from build123d import *

# Parameters (mm, degrees)
F0_R     = 16.51
F1_DEPTH = 50.8
F2_R     = 94.742
F2_R_2   = 75.438
F3_DEPTH = 12.7
F4_R     = 75.438
F5_DEPTH = 31.75
F6_R     = 112.776
F6_R_2   = 69.85
F7_DEPTH = 63.5
F8_R     = 69.85
F9_DEPTH = 76.2


with BuildPart() as f1:
    # F0 (on Top) → F1 (new body)
    with BuildSketch(Plane.XY):
        with BuildLine():
            Line((226.06, 0), (302.641, 0))
            ThreePointArc((302.641, 0), (301.183701, 29.664005), (296.825838, 59.04233))
            Line((296.825838, 59.04233), (34.253926, 6.813529))
            ThreePointArc((34.253926, 6.813529), (34.756827, 3.423249), (34.925, 0))
            Line((34.925, 0), (193.04, 0))
            ThreePointArc((193.04, 0), (209.55, 16.51), (226.06, 0))
        make_face()
        with BuildLine():
            ThreePointArc((0, 302.641), (-213.999503, -213.999503), (302.641, 0))
            Line((302.641, 0), (226.06, 0))
            ThreePointArc((226.06, 0), (209.55, -16.51), (193.04, 0))
            Line((193.04, 0), (34.925, 0))
            ThreePointArc((34.925, 0), (-24.695704, -24.695704), (0, 34.925))
            Line((0, 34.925), (0, 148.59))
            ThreePointArc((0, 148.59), (-16.51, 165.1), (0, 181.61))
            Line((0, 181.61), (0, 232.41))
            ThreePointArc((0, 232.41), (-16.51, 248.92), (0, 265.43))
            Line((0, 265.43), (0, 302.641))
        make_face()
        with Locations((-95.25756, -229.972093)):
            Circle(F0_R, mode=Mode.SUBTRACT)
        with Locations((-63.181035, -152.532511)):
            Circle(F0_R, mode=Mode.SUBTRACT)
        with Locations((-193.598956, -80.191313)):
            Circle(F0_R, mode=Mode.SUBTRACT)
        with Locations((0, -248.92)):
            Circle(F0_R, mode=Mode.SUBTRACT)
        with Locations((95.25756, -229.972093)):
            Circle(F0_R, mode=Mode.SUBTRACT)
        with Locations((0, -165.1)):
            Circle(F0_R, mode=Mode.SUBTRACT)
        with Locations((63.181035, -152.532511)):
            Circle(F0_R, mode=Mode.SUBTRACT)
        with Locations((193.598956, -80.191313)):
            Circle(F0_R, mode=Mode.SUBTRACT)
        with Locations((-209.55, 0)):
            Circle(F0_R, mode=Mode.SUBTRACT)
        with Locations((-193.598956, 80.191313)):
            Circle(F0_R, mode=Mode.SUBTRACT)
        with Locations((-63.181035, 152.532511)):
            Circle(F0_R, mode=Mode.SUBTRACT)
        with Locations((-95.25756, 229.972093)):
            Circle(F0_R, mode=Mode.SUBTRACT)
        with BuildLine():
            Line((34.253926, 6.813529), (296.825838, 59.04233))
            ThreePointArc((296.825838, 59.04233), (213.999503, 213.999503), (59.04233, 296.825838))
            Line((59.04233, 296.825838), (6.813529, 34.253926))
            ThreePointArc((6.813529, 34.253926), (24.695704, 24.695704), (34.253926, 6.813529))
        make_face()
        with Locations((193.598956, 80.191313)):
            Circle(F0_R, mode=Mode.SUBTRACT)
        with Locations((63.181035, 152.532511)):
            Circle(F0_R, mode=Mode.SUBTRACT)
        with Locations((95.25756, 229.972093)):
            Circle(F0_R, mode=Mode.SUBTRACT)
        with BuildLine():
            ThreePointArc((59.04233, 296.825838), (29.664005, 301.183701), (0, 302.641))
            Line((0, 302.641), (0, 265.43))
            ThreePointArc((0, 265.43), (11.674333, 260.594333), (16.51, 248.92))
            ThreePointArc((16.51, 248.92), (11.674333, 237.245667), (0, 232.41))
            Line((0, 232.41), (0, 181.61))
            ThreePointArc((0, 181.61), (11.674333, 176.774333), (16.51, 165.1))
            ThreePointArc((16.51, 165.1), (11.674333, 153.425667), (0, 148.59))
            Line((0, 148.59), (0, 34.925))
            ThreePointArc((0, 34.925), (3.423249, 34.756827), (6.813529, 34.253926))
            Line((6.813529, 34.253926), (59.04233, 296.825838))
        make_face()
    extrude(amount=F1_DEPTH)

    # F2 (on face) → F3 (join)
    with BuildSketch(Plane.XY.offset(50.8)):
        Circle(F2_R)
        Circle(F2_R_2, mode=Mode.SUBTRACT)
    extrude(amount=F3_DEPTH)

    # F4 (on face) → F5 (cut, symmetric)
    with BuildSketch(Plane.XY.offset(63.5)):
        Circle(F4_R)
    extrude(amount=F5_DEPTH, both=True, mode=Mode.SUBTRACT)

    # F6 (on face) → F7 (join)
    with BuildSketch(Plane(origin=(0, 0, 0), x_dir=(1, 0, 0), z_dir=(0, 0, -1))):
        Circle(F6_R)
        Circle(F6_R_2, mode=Mode.SUBTRACT)
    extrude(amount=F7_DEPTH)

    # F8 (on face) → F9 (cut)
    with BuildSketch(Plane(origin=(0, 0, -63.5), x_dir=(1, 0, 0), z_dir=(0, 0, -1))):
        Circle(F8_R)
    extrude(amount=-F9_DEPTH, mode=Mode.SUBTRACT)


solid = f1.part
Can you work these out from the model? Positions are in its coordinate system, mm. A direction names the side the tool comes from. Coordinates: 2 decimals unless noted, no trailing zeros. Order: outer loops, then holes, each group sorted by start corner. A loop starts at its lowest first (then second) coordinate and runs counter-clockwise, first axis right, second up. Notation, with made-up numbers: M 64.25,21 L 72.25,21 A24 ccw 72.25,51 Z; hole C 44.25,20.25 d9. An arc over 180 degrees is marked long. Answer as CSV lines item,"result".
(1) If we mould it in two halves opening along X, with no side actions, what happens to faces 1 (the cylindrical face through (-69.83, 64.03, 57.06)), 2 (the cylindrical face through (193.056, -0.726, 25.044)), 3 (the flat face through (-71, -63, 50.8))? For each: released by +X, released by -X, zero draft, split by the parting line, or undercut.
Geometry check:
face 1,"split by the parting line"
face 2,"undercut"
face 3,"zero draft"
(2) Suppose I cut it at D-D on y = 124.5. Please give me the cut outline in (x, z).
Geometry check:
outline,"M -275.85,0 L 275.85,0 L 275.85,50.8 L -275.85,50.8 Z"
(3) I'm going to push flat-ended pins straight in: pin 1 (12 mm diameter, centred on x = -222, y = 149.5, fed in from -Z); pin 2 (1 mm diameter, centred on x = 43, z = -32, fed in from +Y); pin 3 (10 mm diameter, centred on x = -11.5, y = 25, fed in from -Z); pin 4 (1.5 mm diameter, centred on x = 119.5, z = 16.5, fed in from +Y). Where does each tip first touch, or does it pass through?
Geometry check:
pin 1,"z = 0"
pin 2,"y = 104.46"
pin 3,"through"
pin 4,"y = 278.37"
(4) Please list where these lines run through material, in increasing order: L1, parallel to Y at x = -73, z = 15; L2, parallel to Y at x = 0, z = -37; L3, parallel to X at y = 66, z = 48.
Geometry check:
L1,"-293.7 to -165.81, -139.26 to 139.26, 165.81 to 293.7"
L2,"-112.78 to -69.85, 69.85 to 112.78"
L3,"-295.36 to -202.04, -185.16 to -36.54, 36.54 to 185.16, 202.04 to 295.36"
(5) On a 3-axis mill with a long thin cutter (end or side, diameter ignored), from which of +Z, -Z, +X, -X, +Y, -Y can I reach the whole of each face in a straight line? I mean faces 4 (the flat face through (-4, -130, 0)), 5 (the cylindrical face through (-16.353, -73.644, 47.847)), 6 (the cylindrical face through (301.224, 29.25, 25.044)), 7 (the cylindrical face through (24.49, 24.9, 22.09)). Say none if no direction works.
Geometry check:
face 4,"-Z"
face 5,"+Z"
face 6,"+Z, -Z, +X, +Y"
face 7,"+Z, -Z"
(6) Suppose I cut it at C-C on x = 124. Please give me the cut outline in (y, z), plus the area to 3 significant figures.
Geometry check:
outline,"M -276.07,0 L 276.07,0 L 276.07,50.8 L -276.07,50.8 Z"
area,"28,000 mm^2"
(7) Suppose I cut it at B-B on y = -23.5. Please give me the cut outline in (x, z).
Geometry check:
outline,"M -301.73,0 L -110.3,0 L -110.3,-63.5 L -65.78,-63.5 L -65.78,12.7 L -25.84,12.7 L -25.84,31.75 L -71.68,31.75 L -71.68,63.5 L -91.78,63.5 L -91.78,50.8 L -301.73,50.8 Z; M 25.84,12.7 L 65.78,12.7 L 65.78,-63.5 L 110.3,-63.5 L 110.3,0 L 301.73,0 L 301.73,50.8 L 91.78,50.8 L 91.78,63.5 L 71.68,63.5 L 71.68,31.75 L 25.84,31.75 Z"
(8) Suppose I cut it at A-A on z = -21.5. Please give me the cut outline in (x, y), plus the area to 3 significant figures.
Geometry check:
outline,"C 0,0 d225.55; hole C 0,0 d139.7"
area,"24,600 mm^2"
